Read the model definition and answer for the solid it produces. Units are mm, in the model's axes. Round coordinates to 2 decimals unless told otherwise and drop trailing zeros. Write each loop counter-clockwise with the first axis right and the second up, starting at its lowest first coordinate (ties: lowest second). Pieces come first, ordered by that corner, then holes.
from build123d import *

# Parameters (mm, degrees)
SKETCH5_R           = 3
SKETCH5_W           = 20
SKETCH5_H           = 4
SKETCH5_W_2         = 15
SKETCH5_H_2         = 10
BOSS_EXTRUDE1_DEPTH = 5
SKETCH6_W           = 330
SKETCH6_H           = 15
BOSS_EXTRUDE2_DEPTH = 5
SKETCH8_R           = 2
SKETCH8_R_2         = 3.1
CUT_EXTRUDE1_DEPTH  = 5


with BuildPart() as part:
    # Sketch5 → Boss-Extrude1 (new body)
    with BuildSketch(Plane(origin=(0, 0, 0), x_dir=(0, 0, -1), z_dir=(1, 0, 0))):
        with BuildLine():
            Line((-40, -10), (0, -10))
            Line((0, -10), (0, 0))
            Line((0, 0), (0, 10))
            Line((0, 10), (5, 10))
            Line((5, 10), (5, 0))
            Line((5, 0), (5, -10))
            Line((5, -10), (245, -10))
            Line((245, -10), (245, 0))
            Line((245, 0), (245, 10))
            Line((245, 10), (250, 10))
            Line((250, 10), (250, 0))
            Line((250, 0), (250, -10))
            Line((250, -10), (290, -10))
            Line((290, -10), (290, 50))
            Line((290, 50), (-7.797224701, 50))
            Line((-7.797224701, 50), (-7.797224701, 69.428123594))
            ThreePointArc((-7.797224701, 69.428123594), (-10.726156889, 76.499191405), (-17.797224701, 79.428123594))
            Line((-17.797224701, 79.428123594), (-30, 79.428123594))
            ThreePointArc((-30, 79.428123594), (-37.071067812, 76.499191405), (-40, 69.428123594))
            Line((-40, 69.428123594), (-40, 50))
            Line((-40, 50), (-40, -10))
        make_face()
        with Locations((-25, 35)):
            Circle(SKETCH5_R, mode=Mode.SUBTRACT)
        with Locations((275, 35)):
            Circle(SKETCH5_R, mode=Mode.SUBTRACT)
        with Locations((89.606343961, 42.344097949)):
            Rectangle(SKETCH5_W, SKETCH5_H, mode=Mode.SUBTRACT)
        with Locations((14.606343961, 42.344097949)):
            Rectangle(SKETCH5_W, SKETCH5_H, mode=Mode.SUBTRACT)
        with Locations((-24.047224701, 64.816848726)):
            Rectangle(SKETCH5_W_2, SKETCH5_H_2, mode=Mode.SUBTRACT)
        with Locations((164.606343961, 42.344097949)):
            Rectangle(SKETCH5_W, SKETCH5_H, mode=Mode.SUBTRACT)
        with Locations((239.606343961, 42.344097949)):
            Rectangle(SKETCH5_W, SKETCH5_H, mode=Mode.SUBTRACT)
    extrude(amount=BOSS_EXTRUDE1_DEPTH)

    # Sketch6 → Boss-Extrude2 (add)
    with BuildSketch(Plane(origin=(5, 0, 0), x_dir=(0, 0, -1), z_dir=(1, 0, 0))):
        with Locations((125, -17.5)):
            Rectangle(SKETCH6_W, SKETCH6_H)
    extrude(amount=-BOSS_EXTRUDE2_DEPTH)

    # Sketch8 → Cut-Extrude1 (cut)
    with BuildSketch(Plane(origin=(5, 0, 0), x_dir=(0, 0, -1), z_dir=(1, 0, 0))):
        with Locations((30.968640194, 16)):
            Circle(SKETCH8_R)
        with Locations((30.968640194, -20)):
            Circle(SKETCH8_R)
        with Locations(Location((66.968640194, -20, 0), (0, 0, 180))):
            Circle(SKETCH8_R)
        with Locations(Location((66.968640194, 16, 0), (0, 0, 180))):
            Circle(SKETCH8_R)
        with Locations((48.968640194, -2)):
            Circle(SKETCH8_R_2)
    extrude(amount=-CUT_EXTRUDE1_DEPTH, mode=Mode.SUBTRACT)


solid = part.part
Q1. Section D-D (x = 3.8) is taken. State how many separate pieces and enclosed holes the cut face has, then the cut area to 3 significant figures.
Verdict:
separate pieces: 1
enclosed holes: 14
area: 24,800 mm2
Q2. Section B-B (y = 35) is taken. Determine the outline of the cut face in (x, z).
Verdict:
outline: (0, -290) - (5, -290) - (5, -278) - (0, -278) - close; (0, -272) - (5, -272) - (5, 22) - (0, 22) - close; (0, 28) - (5, 28) - (5, 40) - (0, 40) - close
Q3. Section C-C (y = -2) is taken. Determine the outline of the cut face in (x, z), then the cut area to 3 significant figures.
Verdict:
outline: (0, -290) - (5, -290) - (5, -250) - (0, -250) - close; (0, -245) - (5, -245) - (5, -52.07) - (0, -52.07) - close; (0, -45.87) - (5, -45.87) - (5, -5) - (0, -5) - close; (0, 0) - (5, 0) - (5, 40) - (0, 40) - close
area: 1,570 mm2
Q4. Determine the mould class of faces 1 (the cylindrical face through (2.54, -3.19, -51.83)), 2 (the cylindrical face through (2, 35, -272)), 3 (the flat face through (0, 16, -123)), 4 (the cylindrical face through (2.46, 76.42, 10.65)) for opening direction Y: pulls with the +Y half, pulls with the -Y half, needs draft (parallel to the pull), parting line crosses it, or undercut.
Verdict:
face 1: undercut
face 2: undercut
face 3: needs draft
face 4: pulls with the +Y half
Q5. Flat-ended cylindrical pins translate along their axes: pin 1 Ø1.5 at (x, y) = (2, 58.5) entering from -Z; pin 2 Ø3 at (x, z) = (3, -142.5) entering from +Y. Find the tip coordinate at first contact, or state that the pin passes through.
Verdict:
pin 1: stops at z = 7.8
pin 2: stops at y = 50
Q6. Section A-A (z = -88) is taken. Determine the outline of the cut face in (x, y), then the cut area to 3 significant figures.
Verdict:
outline: (0, -25) - (5, -25) - (5, 40.34) - (0, 40.34) - close; (0, 44.34) - (5, 44.34) - (5, 50) - (0, 50) - close
area: 355 mm2
Q7. Straight lines are drawn through the part: probe 1 along Z at (x, y) = (2.25, -6); probe 2 along Z at (x, y) = (1.25, 35.5); probe 3 along Z at (x, y) = (0.4, 42.5). For each, find the intervals that lie inside material, in ascending order.
Verdict:
probe 1: z = -290 to -250, -245 to -5, 0 to 40
probe 2: z = -290 to -277.96, -272.04 to 22.04, 27.96 to 40
probe 3: z = -290 to -249.61, -229.61 to -174.61, -154.61 to -99.61, -79.61 to -24.61, -4.61 to 40
